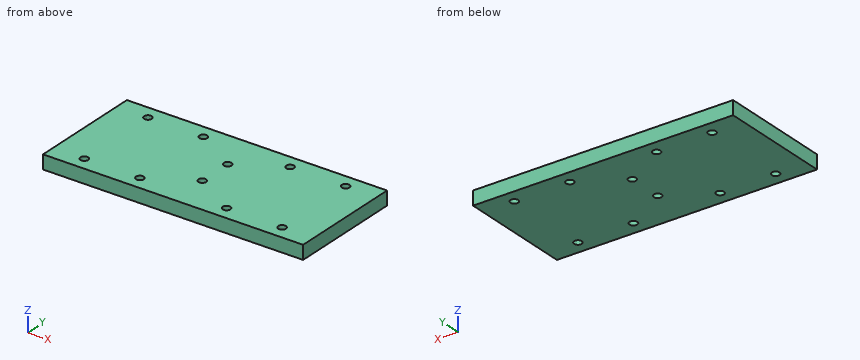
Autodesk Inventor part; units mm, degrees
ref_plane "YZ Plane" through (0, 0, 0) normal (1, 0, 0) x (0, 1, 0)
ref_plane "XZ Plane" through (0, 0, 0) normal (0, 1, 0) x (-1, 0, 0)
ref_plane "XY Plane" through (0, 0, 0) normal (0, 0, 1) x (1, 0, 0)
sketch "Sketch1" plane through (0, 0, 0) normal (0, 0, 1) x (1, 0, 0)
  line L0 (-75, 33) -> (75, 33)
  line L1 (75, 33) -> (75, -33)
  line L2 (75, -33) -> (-75, -33)
  line L3 (-75, -33) -> (-75, 33)
  point P0 (0, 0)
  point P1 (0, 33)
  point P2 (-75, 0)
  dimension "d0" = 150
  dimension "d1" = 66
extrude "Extrusion1" add sketch "Sketch1" along normal blind 8
sketch "Sketch4" plane through (0, 0, 8) normal (0, 0, 1) x (1, 0, 0)
  circle A0 centre (-57, -25) radius 2.25
  circle A1 centre (-57, 25) radius 2.25
  line L0 (-75, 33) -> (-75, -33)
  line L1 (-75, -33) -> (75, -33)
  line L2 (75, 33) -> (-75, 33)
  circle A2 centre (-57, 0) radius 2.25
  circle A3 centre (-25, -25) radius 2.25
  circle A4 centre (-25, 0) radius 2.25
  circle A5 centre (-25, 25) radius 2.25
  circle A6 centre (57, -25) radius 2.25
  line L3 (75, -33) -> (75, 33)
  circle A7 centre (57, 0) radius 2.25
  circle A8 centre (57, 25) radius 2.25
  circle A9 centre (25, -25) radius 2.25
  circle A10 centre (25, 0) radius 2.25
  circle A11 centre (25, 25) radius 2.25
  circle A12 centre (0, -25) radius 2.25
  circle A13 centre (0, 25) radius 2.25
  circle A14 centre (0, 10) radius 2.25
  circle A15 centre (0, -10) radius 2.25
  point P0 (-75, 0)
  point P1 (-75, 0)
  point P2 (0, -33)
  dimension "d19" = 4.5
  dimension "d20" = 18
  dimension "d21" = 8
  dimension "d22" = 8
  dimension "d23" = 32
  dimension "d24" = 18
  dimension "d26" = 32
  dimension "d29" = 10
  dimension "d30" = 10
extrude "Extrusion4" cut sketch "Sketch4" against normal through all contours A0 | A1 | A3 | A5 | A6 | A8 | A9 | A11 | A14 | A15
equation "\"d22\" = d21"
equation "\"d24\" = d20"
equation "\"d26\" = d23"
properties part number "0005-10-012" material "Wood (Maple)"
Here's how the part is built. I have some questions about the finished solid (model axes, mm). Give positions to 0.01 mm unless a question says otherwise; leave off trailing zeros. Write each loop counter-clockwise with the first axis right and the second up, starting at its lowest first coordinate (ties: lowest second). Pieces come first, ordered by that corner, then holes. Notation, with made-up numbers: (84.5, -39.5) -> (108.5, -39.5) arc R11 cw to (108.5, -21.5) -> close; hole circle Ø10 at (32.25, -34.75). An arc over 180 degrees is marked (long way). Write each question's results on one line, items separated by ' | '.
Item 1: Suppose I cut it at C-C on z = 6.5. Give the number of separate pieces and of enclosed holes in the cut face, plus the area to 3 significant figures.
Output:
separate pieces: 1 | enclosed holes: 10 | area: 9,740 mm^2
Item 2: If I drill on L1, parallel to Y at x = 57, z = 4.5; L2, parallel to Y at x = -2, z = 3.25; L3, parallel to X at y = -9, z = 2, over which ranges is the centre line in solid material (lowest first)?
Output:
L1: y = -33 to -27.25, -22.75 to 22.75, 27.25 to 33 | L2: y = -33 to -11.03, -8.97 to 8.97, 11.03 to 33 | L3: x = -75 to -2.02, 2.02 to 75
Item 3: For pin 1 Ø2.5 at (x, y) = (57, 25) entering from +Z, with a flat end and sliding along its axis, tell me the tip position at first contact or that it passes through.
Output:
pin 1: passes through
Item 4: Suppose I cut it at D-D on y = -10. Write out the boundary of the cut face in (x, z).
Output:
outline: (-75, 0) -> (-2.25, 0) -> (-2.25, 8) -> (-75, 8) -> close; (2.25, 0) -> (75, 0) -> (75, 8) -> (2.25, 8) -> close
Item 5: Suppose I cut it at A-A on x = 57. Write out the boundary of the cut face in (y, z).
Output:
outline: (-33, 0) -> (-27.25, 0) -> (-27.25, 8) -> (-33, 8) -> close; (-22.75, 0) -> (22.75, 0) -> (22.75, 8) -> (-22.75, 8) -> close; (27.25, 0) -> (33, 0) -> (33, 8) -> (27.25, 8) -> close
Item 6: Suppose I cut it at B-B on y = -25. Write out the boundary of the cut face in (x, z).
Output:
outline: (-75, 0) -> (-59.25, 0) -> (-59.25, 8) -> (-75, 8) -> close; (-54.75, 0) -> (-27.25, 0) -> (-27.25, 8) -> (-54.75, 8) -> close; (-22.75, 0) -> (22.75, 0) -> (22.75, 8) -> (-22.75, 8) -> close; (27.25, 0) -> (54.75, 0) -> (54.75, 8) -> (27.25, 8) -> close; (59.25, 0) -> (75, 0) -> (75, 8) -> (59.25, 8) -> close
